from build123d import *

# Parameters (mm, degrees)
F0_R     = 10
F1_DEPTH = 10


with BuildPart() as f1:
    # F0 (on Top) → F1 (new body)
    with BuildSketch(Plane.XY):
        with BuildLine():
            ThreePointArc((37.554206, 44.103474), (22.067235, 29.538399), (1.304766, 24.965929))
            ThreePointArc((1.304766, 24.965929), (-19.255297, 15.944702), (-24.284847, -5.93685))
            ThreePointArc((-24.284847, -5.93685), (-9.512511, -33.001447), (16.750607, -49.155795))
            ThreePointArc((16.750607, -49.155795), (39.169931, -41.050494), (37.904534, -17.244596))
            ThreePointArc((37.904534, -17.244596), (36.990811, -9.071889), (44.120823, -4.974213))
            ThreePointArc((44.120823, -4.974213), (51.030762, -3.734261), (56.619703, 0.514089))
            ThreePointArc((56.619703, 0.514089), (65.792763, 16.032989), (69.941986, 33.576228))
            ThreePointArc((69.941986, 33.576228), (57.909572, 51.642912), (37.554206, 44.103474))
        make_face()
        Circle(F0_R, mode=Mode.SUBTRACT)
        with Locations((22.5, -30)):
            Circle(F0_R, mode=Mode.SUBTRACT)
        with Locations((52.5, 35)):
            Circle(F0_R, mode=Mode.SUBTRACT)
    extrude(amount=F1_DEPTH)


solid = f1.part
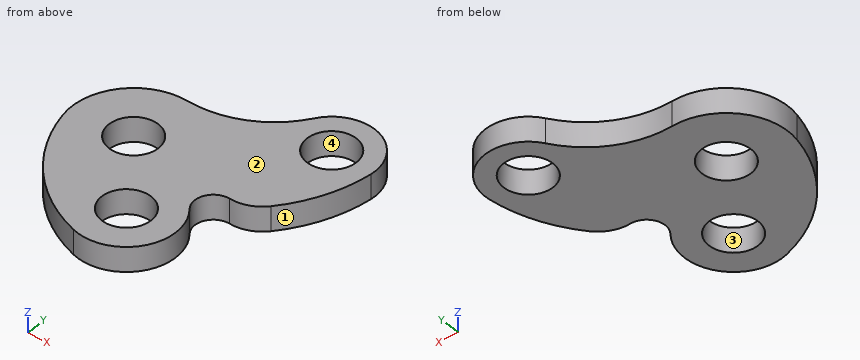
Read the model definition and answer for the solid it produces. Units are mm, in the model's axes. Face numbers are marked on the shaded views. Give positions to 0.01 mm unless a question says otherwise; leave off trailing zeros. Write each loop counter-clockwise with the first axis right and the second up, starting at its lowest first coordinate (ties: lowest second). Pieces come first, ordered by that corner, then holes. Notation, with made-up numbers: (61, 12) -> (92, 12) arc R28 cw to (92, 46) -> close; hole circle Ø10 at (29, -31). An arc over 180 degrees is marked (long way). Answer as a JSON object with one key per item and string values. Group by question number.
1) Find section D-D (y = 22.5). Write down the section's boundary in (x, z), and give its area (3 significant figures).
2) Find section C-C (z = 7.25). Write down the section's boundary in (x, y), and give its area (3 significant figures).
3) The mould has two halves that part along X. Classify the marked faces 1, 2, 3 and 4: +X half, -X half, draft (parallel to the pull), parting line (faces both ways), or undercut.
4) Find section A-A (x = 52.5). Write down the section's boundary in (y, z), and give its area (3 significant figures).
5) Each of these flat-tipped pins is pushed along its axis until it touches: P1, Ø23, axis at x = 52.5, y = 35, coming from the +Z side; P2, Ø2, axis at x = 28.5, z = 3, coming from the +Y side; P3, Ø2, axis at x = 44, z = 8, coming from the -Y side; P4, Ø1, axis at x = 32, z = 8, coming from the -Y side. Where does it stop, or does it pass through?
6) Consider L1, parallel to Y at x = 2.5, z = 4.5; L2, parallel to Y at x = 0, z = 5.75; L3, parallel to X at y = -32.5, z = 9. Determine where each line is inside the solid, lowest interval first. Write a range as from..to.
7) Find section B-B (y = 35). Write down the section's boundary in (x, z), and give its area (4 significant figures).
Values follow:
{
 "1": {"outline": "(-10.9, 0) -> (67.98, 0) -> (67.98, 10) -> (-10.9, 10) -> close", "area": "789 mm2"},
 "2": {"outline": "(-24.28, -5.94) arc R60 ccw to (16.75, -49.16) arc R20 ccw to (37.9, -17.24) arc R7.5 cw to (44.12, -4.97) arc R15 ccw to (56.62, 0.51) arc R60 ccw to (69.94, 33.58) arc R17.5 ccw to (37.55, 44.1) arc R40 cw to (1.3, 24.97) arc R25 ccw to start; hole circle Ø20 at (0, 0); hole circle Ø20 at (22.5, -30); hole circle Ø20 at (52.5, 35)", "area": "4,730 mm2"},
 "3": {"face 1": "+X half", "face 2": "draft", "face 3": "undercut", "face 4": "undercut"},
 "4": {"outline": "(-2.99, 0) -> (25, 0) -> (25, 10) -> (-2.99, 10) -> close; (45, 0) -> (52.5, 0) -> (52.5, 10) -> (45, 10) -> close", "area": "355 mm2"},
 "5": {"P1": "stops at z = 10", "P2": "stops at y = 34.61", "P3": "stops at y = -5", "P4": "stops at y = -47.86"},
 "6": {"L1": "y = -42.76..-9.68, 9.68..24.92", "L2": "y = -41.13..-10, 10..25", "L3": "x = -9.98..12.82, 32.18..42.34"},
 "7": {"outline": "(29.95, 0) -> (42.5, 0) -> (42.5, 10) -> (29.95, 10) -> close; (62.5, 0) -> (70, 0) -> (70, 10) -> (62.5, 10) -> close", "area": "200.5 mm2"}
}
